from build123d import *

# Parameters (mm, degrees)
F2_W = 99.9139621854
F2_H = 95.5784469843
F4_T = 2.54


# Not quite as in the source:
# - the arcs of a loft's sections are written as splines that run evenly, so that the points pair up as in the source's solid
# - a shell that OpenCascade refuses in one call is made with other operations: the cavity is built on its own and cut out


with BuildPart() as f3:
    # F2 (on offset) → F3 section 0
    with BuildSketch(Plane.XY.offset(127)):
        Rectangle(F2_W, F2_H)
    # F0 (on Top) → F3 section 1
    with BuildSketch(Plane.XY):
        with BuildLine():
            add(Edge.make_bspline(
                [(34.2488721695, -32.7627284648), (36.3931877331, -30.5211450231), (38.3166790346, -28.0684255821), (41.6482828465, -22.8347310657), (43.0563129764, -20.0538854036), (45.3028578067, -14.2707911992), (46.1413169567, -11.2686856553), (47.2164693474, -5.1584328302), (47.4531360028, -2.0504366369), (47.3155784505, 4.1521612197), (46.9413576443, 7.2466095116), (45.5963764086, 13.3031900424), (44.6256492365, 16.2651725205), (42.1249311921, 21.9429847323), (40.5950021549, 24.658674071), (37.0346484938, 29.7395228248), (35.0043119065, 32.1045566058), (32.7627284648, 34.2488721695)],
                knots=[0, 0, 0, 0, 0.125, 0.125, 0.25, 0.25, 0.375, 0.375, 0.5, 0.5, 0.625, 0.625, 0.75, 0.75, 0.875, 0.875, 1, 1, 1, 1], degree=3))
            add(Edge.make_bspline(
                [(32.7627284648, 34.2488721695), (30.5211450231, 36.3931877331), (28.0684255821, 38.3166790346), (22.8347310657, 41.6482828465), (20.0538854036, 43.0563129764), (14.2707911992, 45.3028578067), (11.2686856553, 46.1413169567), (5.1584328302, 47.2164693474), (2.0504366369, 47.4531360028), (-4.1521612197, 47.3155784505), (-7.2466095116, 46.9413576443), (-13.3031900424, 45.5963764086), (-16.2651725205, 44.6256492365), (-21.9429847323, 42.1249311921), (-24.658674071, 40.5950021549), (-29.7395228248, 37.0346484938), (-32.1045566058, 35.0043119065), (-34.2488721695, 32.7627284648)],
                knots=[0, 0, 0, 0, 0.125, 0.125, 0.25, 0.25, 0.375, 0.375, 0.5, 0.5, 0.625, 0.625, 0.75, 0.75, 0.875, 0.875, 1, 1, 1, 1], degree=3))
            add(Edge.make_bspline(
                [(-34.2488721695, 32.7627284648), (-36.3931877331, 30.5211450231), (-38.3166790346, 28.0684255821), (-41.6482828465, 22.8347310657), (-43.0563129764, 20.0538854036), (-45.3028578067, 14.2707911992), (-46.1413169567, 11.2686856553), (-47.2164693474, 5.1584328302), (-47.4531360028, 2.0504366369), (-47.3155784505, -4.1521612197), (-46.9413576443, -7.2466095116), (-45.5963764086, -13.3031900424), (-44.6256492365, -16.2651725205), (-42.1249311921, -21.9429847323), (-40.5950021549, -24.658674071), (-37.0346484938, -29.7395228248), (-35.0043119065, -32.1045566058), (-32.7627284648, -34.2488721695)],
                knots=[0, 0, 0, 0, 0.125, 0.125, 0.25, 0.25, 0.375, 0.375, 0.5, 0.5, 0.625, 0.625, 0.75, 0.75, 0.875, 0.875, 1, 1, 1, 1], degree=3))
            add(Edge.make_bspline(
                [(-32.7627284648, -34.2488721695), (-30.5211450231, -36.3931877331), (-28.0684255821, -38.3166790346), (-22.8347310657, -41.6482828465), (-20.0538854036, -43.0563129764), (-14.2707911992, -45.3028578067), (-11.2686856553, -46.1413169567), (-5.1584328302, -47.2164693474), (-2.0504366369, -47.4531360028), (4.1521612197, -47.3155784505), (7.2466095116, -46.9413576443), (13.3031900424, -45.5963764086), (16.2651725205, -44.6256492365), (21.9429847323, -42.1249311921), (24.658674071, -40.5950021549), (29.7395228248, -37.0346484938), (32.1045566058, -35.0043119065), (34.2488721695, -32.7627284648)],
                knots=[0, 0, 0, 0, 0.125, 0.125, 0.25, 0.25, 0.375, 0.375, 0.5, 0.5, 0.625, 0.625, 0.75, 0.75, 0.875, 0.875, 1, 1, 1, 1], degree=3))
        make_face()
    loft(ruled=True)

    # F4: shell of thickness 2.54, made by hand


with BuildPart() as f4_core1:
    # F4_t2: copy of F3
    add(f3.part)

    # the walls: a layer under each face that stays
    f4_faces = [f4_core1.faces().sort_by_distance(p)[0] for p in [
        (0.5254311457, -47.5867903594, 63.5),
        (48.6706691597, 0.5254311457, 63.5),
        (-0.5254311457, 47.5867903594, 63.5),
        (-48.6706691597, -0.5254311457, 63.5),
        (0, 0, 0),
    ]]
    thicken(f4_faces, amount=-F4_T, mode=Mode.SUBTRACT)


with BuildPart() as f3_1:
    add(f3.part)

    # what is left inside the walls is the cavity
    f4_cavity = [f4_core1.part.solids().sort_by_distance(p)[0] for p in [
        (0.329341, -45.091155, 85.374003),
    ]]
    add(f4_cavity, mode=Mode.SUBTRACT)


solid = f3_1.part
Geometry: final body of the model. Coordinates: model frame, mm. Round coordinates to 2 decimals unless told otherwise and drop trailing zeros. Write each question's results on one line, items separated by ' | '. Start each with the question number.
1) Mould query, pull axis X, two halves, no side actions, for faces 1 (the face through (2, -47, 127)), 2 (the face through (-1, 0, 2.54)). Classes: released by +X, released by -X, zero draft, split by the parting line, or undercut.
2) Line query: probe 1 along X at (y, z) = (8, 61); probe 2 along Y at (x, z) = (-26.5, 108); probe 3 along Y at (x, z) = (1, 108). Output: solid intervals per line, ascending. Write a range as [from, to].
3) First-contact query: P1, Ø12, axis at x = 19, y = 12, coming from the +Z side; P2, Ø2, axis at x = 6, z = 79.5, coming from the -Y side; P3, Ø4, axis at y = -22.5, z = 58.5, coming from the -X side. Flat tips, straight axial feed; report the tip coordinate or a pass-through.
Verdict:
1) face 1: zero draft | face 2: undercut
2) probe 1: x = [-48.4, -45.85], [45.76, 48.31] | probe 2: y = [-47.13, -44.58], [44.46, 47.01] | probe 3: y = [-47.73, -45.19], [45.19, 47.73]
3) P1: stops at z = 2.54 | P2: stops at y = -47.55 | P3: stops at x = -46.58
